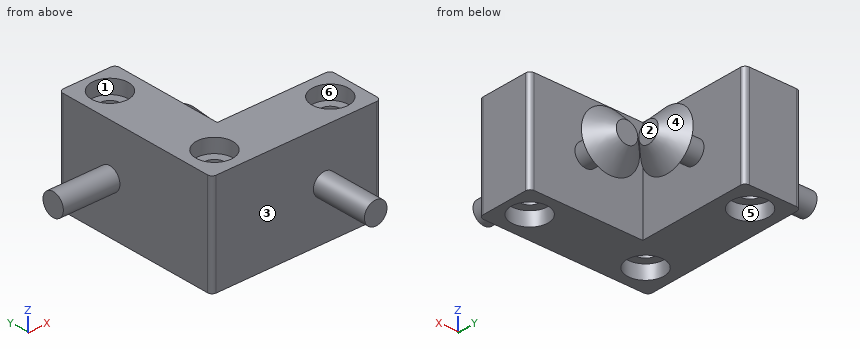
from build123d import *

# Parameters (mm, degrees)
BOSS_EXTRUDE2_DEPTH = 18
SKETCH2_R           = 1.75
CUT_EXTRUDE1_DEPTH  = 18
SKETCH3_R           = 3.25
CUT_EXTRUDE2_DEPTH  = 2.5
FILLET1_R           = 0.8
SKETCH4_R           = 2
BOSS_EXTRUDE3_DEPTH = 10


with BuildPart() as part:
    # Sketch1 → Boss-Extrude2 (new body)
    with BuildSketch(Plane.XY):
        Polygon((0, 0), (0, 30), (10, 30), (10, 10), (30, 10), (30, 0), align=None)
    extrude(amount=BOSS_EXTRUDE2_DEPTH)

    # Sketch2 → Cut-Extrude1 (cut)
    with BuildSketch(Plane(origin=(0, 0, 0), x_dir=(-1, 0, 0), z_dir=(0, 0, -1))):
        with Locations((-25.5, 5)):
            Circle(SKETCH2_R)
        with Locations((-5, 5)):
            Circle(SKETCH2_R)
        with Locations((-5, 25.5)):
            Circle(SKETCH2_R)
    extrude(amount=-CUT_EXTRUDE1_DEPTH, mode=Mode.SUBTRACT)

    # Sketch3 → Cut-Extrude2 (cut)
    with BuildSketch(Plane(origin=(0, 0, 0), x_dir=(-1, 0, 0), z_dir=(0, 0, -1))):
        with Locations((-25.5, 5)):
            Circle(SKETCH3_R)
        with Locations((-5, 5)):
            Circle(SKETCH3_R)
        with Locations((-5, 25.5)):
            Circle(SKETCH3_R)
    cut_extrude2 = extrude(amount=-CUT_EXTRUDE2_DEPTH, mode=Mode.SUBTRACT)

    # Mirror1: Cut-Extrude2 across plane
    add(cut_extrude2.mirror(Plane.XY.offset(9)), mode=Mode.SUBTRACT)

    # Fillet1
    fillet1_edges = [part.edges().sort_by_distance(p)[0] for p in [
        (10, 30, 9),
        (0, 30, 9),
        (0, 0, 9),
        (30, 0, 9),
        (30, 10, 9),
    ]]
    fillet(fillet1_edges, radius=FILLET1_R)

    # Sketch4 → Boss-Extrude3 (add)
    with BuildSketch(Plane.XZ):
        with Locations(Location((20, 9, 0), (0, 0, 270))):
            Circle(SKETCH4_R)
    boss_extrude3 = extrude(amount=BOSS_EXTRUDE3_DEPTH)

    # Mirror2: Boss-Extrude3 across plane
    add(boss_extrude3.mirror(Plane(origin=(0, 0, 0), x_dir=(0, 0, 1), z_dir=(0.7071067811865438, -0.7071067811865512, 0))))

    # Sketch5 → Revolve4 (revolve)
    with BuildSketch(Plane.XY.offset(9), mode=Mode.PRIVATE) as revolve4_sk:
        Polygon((18, 10), (18, 14.752860349), (14.85, 14.752860349), (18.097139651, 18), (20, 18), (20, 10), align=None)
    revolve4 = revolve(revolve4_sk.sketch.rotate(Axis((20, 23.873341049, 9), (0, -1, 0)), 270), axis=Axis((20, 23.873341049, 9), (0, -1, 0)))

    # Mirror7: Revolve4 across plane
    add(revolve4.mirror(Plane(origin=(0, 0, 0), x_dir=(0, 0, 1), z_dir=(0.7071067811865438, -0.7071067811865512, 0))))


solid = part.part
Input: part model. Units: mm. Frame: model coordinates. Face numbers are marked on the shaded views. A direction names the side the tool comes from. Give positions to 0.01 mm unless a question says otherwise; leave off trailing zeros. Write each loop counter-clockwise with the first axis right and the second up, starting at its lowest first coordinate (ties: lowest second). Pieces come first, ordered by that corner, then holes. Notation, with made-up numbers: (-11, 8) -> (45, 8) arc R28 ccw to (45, 37) -> close; hole circle Ø10 at (85.25, 67.25). An arc over 180 degrees is marked (long way). Use one line per item in the form item = value. Start each with the question number.
1) Section query C-C on z = 15. Return the cut outline in (x, y), then the cut area to 3 significant figures.
2) Ray query, probe 1 along Y at (x, z) = (5, 1.55); probe 2 along Y at (x, z) = (25.5, 17); probe 3 along X at (y, z) = (11.5, 5). Return the intervals inside material, ascending. Write a range as from..to.
3) Set-up query: the marked faces 4, 5 and 6. Return all of +Z, -Z, +X, -X, +Y, -Y with unobstructed straight access to the full face (end or side cutting, diameter ignored); none if empty.
4) Pin query (flat end, axial travel): pin 1 (5 mm diameter, centred on x = 5, y = 4.5, fed in from +Z); pin 2 (3 mm diameter, centred on x = 1, z = 8.5, fed in from -Y); pin 3 (1.5 mm diameter, centred on x = -0.5, z = 12.5, fed in from -Y). Return the tip coordinate at first contact, or that it passes through.
5) Section query A-A on y = 5. Return the cut outline in (x, z), then the cut area to 3 significant figures.
6) Draft query along Y for the marked faces 1, 2 and 3. Return one class per face: pulls with the +Y half, pulls with the -Y half, needs draft (parallel to the pull), parting line crosses it, or undercut.
7) Section query D-D on x = 20. Return the cut outline in (y, z), then the cut area to 3 significant figures.
Outcome:
q1.outline = (0, 0.8) arc R0.8 ccw to (0.8, 0) -> (29.2, 0) arc R0.8 ccw to (30, 0.8) -> (30, 9.2) arc R0.8 ccw to (29.2, 10) -> (10, 10) -> (10, 29.2) arc R0.8 ccw to (9.2, 30) -> (0.8, 30) arc R0.8 ccw to (0, 29.2) -> close; hole circle Ø3.5 at (5, 5); hole circle Ø3.5 at (5, 25.5); hole circle Ø3.5 at (25.5, 5)
q1.area = 470 mm^2
q2.probe_1 = 0..1.75, 8.25..22.25, 28.75..30
q2.probe_2 = 0..1.75, 8.25..10
q2.probe_3 = 0..10
q3.face_4 = none
q3.face_5 = -Z
q3.face_6 = +Z
q4.pin_1 = 15.5
q4.pin_2 = 0
q4.pin_3 = 0.22
q5.outline = (0, 0) -> (1.75, 0) -> (1.75, 2.5) -> (3.25, 2.5) -> (3.25, 15.5) -> (1.75, 15.5) -> (1.75, 18) -> (0, 18) -> close; (6.75, 2.5) -> (8.25, 2.5) -> (8.25, 0) -> (22.25, 0) -> (22.25, 2.5) -> (23.75, 2.5) -> (23.75, 15.5) -> (22.25, 15.5) -> (22.25, 18) -> (8.25, 18) -> (8.25, 15.5) -> (6.75, 15.5) -> close; (27.25, 2.5) -> (28.75, 2.5) -> (28.75, 0) -> (30, 0) -> (30, 18) -> (28.75, 18) -> (28.75, 15.5) -> (27.25, 15.5) -> close
q5.area = 384 mm^2
q6.face_1 = undercut
q6.face_2 = needs draft
q6.face_3 = pulls with the -Y half
q7.outline = (-10, 7) -> (0, 7) -> (0, 0) -> (10, 0) -> (10, 7) -> (14.75, 7) -> (14.75, 3.85) -> (18, 7.1) -> (18, 10.9) -> (14.75, 14.15) -> (14.75, 11) -> (10, 11) -> (10, 18) -> (0, 18) -> (0, 11) -> (-10, 11) -> close
q7.area = 262 mm^2
